The model under review builds one solid part; all positions refer to its coordinate system, in mm. Coordinates: 2 decimals unless noted, no trailing zeros. Use one line per item in the form item = value.
```python
from build123d import *

# Parameters (mm, degrees)
F0_W     = 203.2
F0_H     = 101.6
F1_DEPTH = 12.7
F2_R     = 9.525
F4_D     = 4.7752
F6_D     = 6.35


with BuildPart() as f1:
    # F0 (on Front) → F1 (new body)
    with BuildSketch(Plane.XZ):
        with Locations((-0.184152, 17.884531)):
            Rectangle(F0_W, F0_H)
    extrude(amount=F1_DEPTH)

    # F2
    f2_edges = [f1.edges().sort_by_distance(p)[0] for p in [
        (-101.784152, -6.35, 68.684531),
        (101.415848, -6.35, 68.684531),
        (101.415848, -6.35, -32.915469),
        (-101.784152, -6.35, -32.915469),
    ]]
    fillet(f2_edges, radius=F2_R)

    # F4 (through all)
    with Locations(Plane.XZ.offset(12.7)):
        with Locations((-89.084152, 55.984531), (-89.084152, -20.215469), (88.715848, -20.215469), (88.715848, 55.984531)):
            Hole(F4_D / 2)

    # F6 (through all)
    with Locations(Plane.XZ.offset(12.7)):
        with Locations((-63.684152, 30.584531), (-63.684152, 5.184531), (63.315848, 5.184531), (63.315848, 30.584531)):
            Hole(F6_D / 2)


solid = f1.part
```
1. The part is to be moulded in two halves that separate along Z. For faces 1 (the face through (-91.3, -6.3, -21.1)), 2 (the face through (-99.07, -6.44, -30.05)), 3 (the face through (86.5, -6.3, 55.1)), 4 (the face through (-2, 0, 19)), say which applies: pulls with the +Z half, pulls with the -Z half, needs draft (parallel to the pull), parting line crosses it, or undercut.
Response values:
face_1 = undercut
face_2 = pulls with the -Z half
face_3 = undercut
face_4 = needs draft
2. Insertion check: P1, Ø4, axis at x = 27.5, z = -22, coming from the +Y side. The pin has a flat end and moves straight along its axis. Give the tip position at first contact, or say it passes through.
Response values:
P1 = 0
3. Wall thickness on line 1 along X through (y, z) = (-1.75, -20); line 2 along Z through (x, y) = (65, -11.5); line 3 along X through (y, z) = (-0.25, 55.5): over which ranges is each line inside the solid? List them lowest first. Write a range as from..to.
Response values:
line_1 = -101.78..-91.46, -86.71..86.34, 91.09..101.42
line_2 = -32.92..2.49, 7.88..27.89, 33.28..68.68
line_3 = -101.78..-91.42, -86.75..86.38, 91.05..101.42
